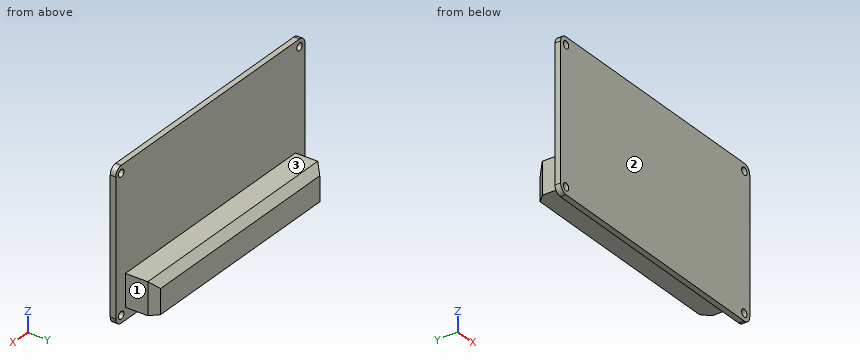
from build123d import *

# Parameters (mm, degrees)
SKETCH1_W           = 70
SKETCH1_H           = 40
BOSS_EXTRUDE1_DEPTH = 1.5
SKETCH2_W           = 62.906558998
SKETCH2_H           = 8.609060895
BOSS_EXTRUDE2_DEPTH = 8
CHAMFER1_SIZE       = 2
SKETCH3_R           = 1
CUT_EXTRUDE1_DEPTH  = 42.097445176
FILLET1_R           = 2


with BuildPart() as part:
    # Sketch1 → Boss-Extrude1 (new body)
    with BuildSketch(Plane(origin=(0, 0, 0), x_dir=(1, 0, 0), z_dir=(0, 1, 0))):
        Rectangle(SKETCH1_W, SKETCH1_H)
    extrude(amount=BOSS_EXTRUDE1_DEPTH)

    # Sketch2 → Boss-Extrude2 (add)
    with BuildSketch(Plane(origin=(0, 1.5, 0), x_dir=(1, 0, 0), z_dir=(0, 1, 0))):
        with Locations((0, 12.448226713)):
            Rectangle(SKETCH2_W, SKETCH2_H)
    extrude(amount=BOSS_EXTRUDE2_DEPTH)

    # Chamfer1
    chamfer1_edges = [part.edges().sort_by_distance(p)[0] for p in [
        (31.453279499, 9.5, -12.448226713),
        (-31.453279499, 9.5, -12.448226713),
        (0, 9.5, -8.143696265),
    ]]
    chamfer(chamfer1_edges, length=CHAMFER1_SIZE)

    # Sketch3 → Cut-Extrude1 (cut, through all)
    with BuildSketch(Plane(origin=(0, 1.5, 0), x_dir=(1, 0, 0), z_dir=(0, 1, 0))):
        with Locations(Location((-33, -18, 0), (0, 0, 270))):
            Circle(SKETCH3_R)
        with Locations(Location((-33, 18, 0), (0, 0, 270))):
            Circle(SKETCH3_R)
        with Locations(Location((33, 18, 0), (0, 0, 270))):
            Circle(SKETCH3_R)
        with Locations(Location((33, -18, 0), (0, 0, 270))):
            Circle(SKETCH3_R)
    extrude(amount=-CUT_EXTRUDE1_DEPTH, mode=Mode.SUBTRACT)

    # Fillet1
    fillet1_edges = [part.edges().sort_by_distance(p)[0] for p in [
        (35, 0.75, 20),
        (-35, 0.75, 20),
        (-35, 0.75, -20),
        (35, 0.75, -20),
    ]]
    fillet(fillet1_edges, radius=FILLET1_R)


solid = part.part
Input: part model. Units: mm. Frame: model coordinates. Face numbers are marked on the shaded views. A direction names the side the tool comes from. Give positions to 0.01 mm unless a question says otherwise; leave off trailing zeros. Order: outer loops, then holes, each group sorted by start corner. A loop starts at its lowest first (then second) coordinate and runs counter-clockwise, first axis right, second up. Notation, with made-up numbers: (38.5, 40.5) - (74.5, 40.5) arc R19 ccw to (74.5, 68.5) - close; hole circle Ø4 at (14, 5.5). An arc over 180 degrees is marked (long way). Write each question's results on one line, items separated by ' | '.
Item 1: Section D-D (z = -2). Return loops of the section in (x, y), and give its area (3 significant figures).
A:
outline: (-35, 0) - (35, 0) - (35, 1.5) - (-35, 1.5) - close | area: 105 mm^2
Item 2: Access query for the marked faces 1, 2 and 3. Directions: +Z, -Z, +X, -X, +Y, -Y. A direction counts if a zero-diameter tool reaches every point of the face in a straight line with its end or side. Return the directions, or none.
A:
face 1: +Z, -Z, +X, +Y | face 2: +Z, -Z, +X, -X, -Y | face 3: +Z, +X, -X, +Y
Item 3: Section A-A (z = -13). Return loops of the section in (x, y), and give its area (3 significant figures).
A:
outline: (-35, 0) - (35, 0) - (35, 1.5) - (31.45, 1.5) - (31.45, 7.5) - (29.45, 9.5) - (-29.45, 9.5) - (-31.45, 7.5) - (-31.45, 1.5) - (-35, 1.5) - close | area: 604 mm^2
Item 4: Section B-B (x = 19.5). Return loops of the section in (y, z), and give its area (3 significant figures).
A:
outline: (0, -20) - (1.5, -20) - (1.5, -16.75) - (9.5, -16.75) - (9.5, -10.14) - (7.5, -8.14) - (1.5, -8.14) - (1.5, 20) - (0, 20) - close | area: 127 mm^2
Item 5: Section C-C (y = 5). Return loops of the section in (x, z), and give its area (3 significant figures).
A:
outline: (-31.45, -16.75) - (31.45, -16.75) - (31.45, -8.14) - (-31.45, -8.14) - close | area: 542 mm^2
Item 6: Material intervals for line 1 along X through (y, z) = (1.05, -18); line 2 along Y through (x, z) = (-2.5, -7); line 3 along Z through (x, y) = (10.5, 4.5), sorted ascending.
A:
line 1: x = -35 to -34, -32 to 32, 34 to 35 | line 2: y = 0 to 1.5 | line 3: z = -16.75 to -8.14
Item 7: Contact query for flat-ended pins moving along their axis: pin 1 Ø2.5 at (x, z) = (-33, 18) entering from +Y; pin 2 Ø1.8 at (x, y) = (9.5, 3.5) entering from +Z; pin 3 Ø3 at (y, z) = (6, -11) entering from +X; pin 4 Ø1.2 at (x, z) = (33, -18) entering from +Y. Output: stop coordinate, or through.
A:
pin 1: stops at y = 1.5 | pin 2: stops at z = -8.14 | pin 3: stops at x = 31.45 | pin 4: passes through
